Check sheet for the modelled part. Datum: model origin and axes. Units: mm. A direction names the side the tool comes from. Give positions to 0.01 mm unless a question says otherwise; leave off trailing zeros. Loops run counter-clockwise (first coordinate to the right, second up) from the corner with the lowest first, then second, coordinate; pieces in that order, holes last. Notation, with made-up numbers: M 61.5,83.5 L 111.5,83.5 A17 cw 111.5,102.5 Z; hole C -34,-40 d7. An arc over 180 degrees is marked long. Put each result on its own line as item: value. Start each with the question number.
```python
from build123d import *
from OCP.BRepFilletAPI import BRepFilletAPI_MakeFillet

# Parameters (mm, degrees)
SKETCH1_R           = 25.75
BOSS_EXTRUDE1_DEPTH = 25
SKETCH2_R           = 20.5
SKETCH2_R_2         = 8
BOSS_EXTRUDE2_DEPTH = 5
BOSS_EXTRUDE3_DEPTH = 50
SKETCH5_R           = 8
CUT_EXTRUDE1_DEPTH  = 1086.176840005
SKETCH6_R           = 17.5
CUT_EXTRUDE2_DEPTH  = 15
SKETCH7_W           = 8
SKETCH7_H           = 9
CUT_EXTRUDE3_DEPTH  = 35
BOSS_EXTRUDE4_DEPTH = 40
SKETCH9_R           = 6
CUT_EXTRUDE4_DEPTH  = 38.2
FILLET1_R1          = 20
FILLET1_R2          = 10


with BuildPart() as part:
    # Sketch1 → Boss-Extrude1 (new, symmetric)
    with BuildSketch(Plane.XY):
        with BuildLine():
            Line((0, 0), (-25, 0))
            Line((-25, 0), (-25, 110))
            Line((-25, 110), (145, 110))
            Line((145, 110), (145, 28.867513459))
            Line((145, 28.867513459), (474.063730334, 218.852546748))
            ThreePointArc((474.063730334, 218.852546748), (510.873444118, 277.555083571), (567.103024177, 237.06833037))
            Line((567.103024177, 237.06833037), (983.374527569, 163.668433022))
            ThreePointArc((983.374527569, 163.668433022), (1022.625735123, 177.590092488), (1047.403876506, 144.116018842))
            Line((1047.403876506, 144.116018842), (1047.403876506, 84.116018842))
            Line((1047.403876506, 84.116018842), (978.437892023, 84.116018842))
            Line((978.437892023, 84.116018842), (978.437892023, 135.671381603))
            Line((978.437892023, 135.671381603), (562.166388631, 209.071278951))
            ThreePointArc((562.166388631, 209.071278951), (527.367103522, 184.014892858), (486.563730334, 197.201911654))
            Line((486.563730334, 197.201911654), (145, 0))
            Line((145, 0), (120, 0))
            Line((120, 0), (120, 85))
            Line((120, 85), (0, 85))
            Line((0, 85), (0, 0))
        make_face()
        with Locations((520, 230.940107676)):
            Circle(SKETCH1_R, mode=Mode.SUBTRACT)
    extrude(amount=BOSS_EXTRUDE1_DEPTH, both=True)

    # Sketch2 → Boss-Extrude2 (add)
    with BuildSketch(Plane.XY.offset(-25)):
        with Locations((1012.403876506, 144.116018842)):
            Circle(SKETCH2_R)
        with Locations((1012.403876506, 144.116018842)):
            Circle(SKETCH2_R_2, mode=Mode.SUBTRACT)
    extrude(amount=-BOSS_EXTRUDE2_DEPTH)

    # Sketch4 → Boss-Extrude3 (add)
    with BuildSketch(Plane.XY.offset(25)):
        Polygon((145, 110), (347.313653274, 145.673355638), (309.33231998, 123.744822637), (145, 94.768600822), align=None)
    extrude(amount=-BOSS_EXTRUDE3_DEPTH)

    # Sketch5 → Cut-Extrude1 (cut, through all)
    with BuildSketch(Plane.XY.offset(25)):
        with Locations((1012.403876506, 144.116018842)):
            Circle(SKETCH5_R)
    extrude(amount=-CUT_EXTRUDE1_DEPTH, mode=Mode.SUBTRACT)

    # Sketch6 → Cut-Extrude2 (cut)
    with BuildSketch(Plane(origin=(0, 0, 25), x_dir=(-1, 0, 0), z_dir=(0, 0, -1))):
        with Locations((-1012.403876506, 144.116018842)):
            Circle(SKETCH6_R)
    extrude(amount=CUT_EXTRUDE2_DEPTH, mode=Mode.SUBTRACT)

    # Sketch7 → Cut-Extrude3 (cut)
    with BuildSketch(Plane.XY.offset(-25)):
        Polygon((120, 85), (145, 85), (145, 70), (120, 45), align=None)
        Polygon((347.313653274, 145.673355638), (309.33231998, 123.744822637), (283.417852806, 119.175402883), (321.3991861, 141.103935884), align=None)
        with Locations((-4, 67.5)):
            Rectangle(SKETCH7_W, SKETCH7_H)
    extrude(amount=CUT_EXTRUDE3_DEPTH, mode=Mode.SUBTRACT)

    # Sketch8 → Boss-Extrude4 (add)
    with BuildSketch(Plane.XY.offset(-25)):
        Polygon((991.153876506, 84.116018842), (1033.653876506, 84.116018842), (1019.903876506, 104.116018842), (1004.903876506, 104.116018842), align=None)
    extrude(amount=-BOSS_EXTRUDE4_DEPTH)

    # Sketch9 → Cut-Extrude4 (cut)
    with BuildSketch(Plane.XZ):
        with Locations((-7.475, 0)):
            Circle(SKETCH9_R)
        with Locations((127.475, 0)):
            Circle(SKETCH9_R)
    extrude(amount=-CUT_EXTRUDE4_DEPTH, mode=Mode.SUBTRACT)

    # Fillet1: one fillet with a radius per group of edges: ONE call of the kernel's fillet builder (fillet() takes one radius for all edges)
    fillet1_edges_1 = [part.edges().sort_by_distance(p)[0] for p in [
        (-25, 110, 0),
    ]]
    fillet1_edges_2 = [part.edges().sort_by_distance(p)[0] for p in [
        (1047.403876506, 84.116018842, 0),
        (978.437892023, 84.116018842, 0),
    ]]
    fillet1 = BRepFilletAPI_MakeFillet(part.part.solid().wrapped)
    for e in fillet1_edges_1:
        fillet1.Add(FILLET1_R1, e.wrapped)
    for e in fillet1_edges_2:
        fillet1.Add(FILLET1_R2, e.wrapped)
    add(Compound.cast(fillet1.Shape()), mode=Mode.REPLACE)


solid = part.part
```
Q1. Depth check by flat-ended pin: P1, Ø7, axis at x = -7.475, z = 0, coming from the -Y side; P2, Ø9.5, axis at x = 127.475, z = 0, coming from the +Y side; P3, Ø21, axis at y = 105, z = 3.5, coming from the -X side. Enter the tip coordinate at first touch or a pass-through.
Q2. Thickness scan on line 1 along Y through (x, z) = (514, 6); line 2 along Z through (x, y) = (441, 178); line 3 along Y through (x, z) = (63, 2). Record the ranges inside material, lowest first. Write a range as [from, to].
Q3. Section check A-A, the plane x = 520. Record the cut outline in (y, z).
Q4. Access from +Z, -Z, +X, -X, +Y, -Y to the whole of each face (thin tool, end or side, straight path). Record for faces 1 (the face through (772.325, 200.882, 0.35)), 2 (the face through (1013, 84.116, -19)), 3 (the face through (0, 43, 0)).
Q5. Section check D-D, the plane x = 849.5. Record the cut outline in (y, z).
Q6. Section check C-C, the plane x = 181.5. Record the cut outline in (y, z).
Q7. Mould release check, pull along Y, two halves, no side actions. Record for faces 4 (the face through (978.438, 115, 0)), 5 (the face through (130, 70, 10)), 6 (the face through (-18.986, 104.297, -0.35)): pulls with the +Y half, pulls with the -Y half, needs draft (parallel to the pull), parting line crosses it, or undercut.
Q8. Section check B-B, the plane z = -49. Record the cut outline in (x, y), then the cut area to 3 significant figures.
Found:
1. P1: stops at y = 38.2
1. P2: stops at y = 110
1. P3: stops at x = -24.49
2. line 1: y = [183.82, 205.9], [255.98, 278.06]
2. line 2: z = [-25, 25]
2. line 3: y = [85, 110]
3. outline: M 183.44,-25 L 205.19,-25 L 205.19,25 L 183.44,25 Z; M 256.69,-25 L 278.44,-25 L 278.44,25 L 256.69,25 Z
4. face 1: +Z, -Z, +Y
4. face 2: +Z, -Z, +X, -Y
4. face 3: +Z, -Z, -Y
5. outline: M 158.41,-25 L 187.27,-25 L 187.27,25 L 158.41,25 Z
6. outline: M 21.07,-25 L 49.94,-25 L 49.94,25 L 21.07,25 Z; M 101.2,-25 L 116.44,-25 L 116.44,25 L 101.2,25 Z
7. face 4: needs draft
7. face 5: undercut
7. face 6: pulls with the +Y half
8. outline: M 991.15,84.12 L 1033.65,84.12 L 1019.9,104.12 L 1004.9,104.12 Z
8. area: 575 mm^2
